The model under review builds one solid part; all positions refer to its coordinate system, in mm. Coordinates: 2 decimals unless noted, no trailing zeros. Order: outer loops, then holes, each group sorted by start corner. A loop starts at its lowest first (then second) coordinate and runs counter-clockwise, first axis right, second up. Notation, with made-up numbers: (66.5, -31) -> (104.5, -31) arc R13 cw to (104.5, -25) -> close; hole circle Ø3 at (18, -21.5). An arc over 180 degrees is marked (long way). Use one line per item in the form item = value. Start each with the question number.
(1) Take a section at A-A (z = 38). State the section outline as (x, y) points.
(2) Take a section at C-C (x = 4.75). State the section outline as (y, z) points, then the cut area to 3 significant figures.
(3) Insertion check: pin 1 Ø4 at (y, z) = (22.5, 85.5) entering from +X; pin 2 Ø2 at (x, y) = (4, -38.5) entering from -Z. Each pin has a flat end and moves straight along its axis. Give the tip position at first contact, or say it passes through.
(4) Take a section at B-B (y = -4.5). State the section outline as (x, z) points.
(5) Wall thickness on line 1 along X through (y, z) = (39.5, 91); line 2 along Z through (x, y) = (4, 18); line 3 along Z through (x, y) = (4.25, 23): over which ranges is each line inside the solid? List them lowest first.
```python
from build123d import *

# Parameters (mm, degrees)
F0_W        = 4.0632686578
F0_H        = 96.9379618764
F1_DEPTH    = 121
F2_W        = 94.1168889403
F2_H        = 118.3094680309
F3_DEPTH    = 0.2
F4_W        = 84.7520232201
F4_H        = 13.4229809046
F5_DEPTH    = 4.2
F6_T1_DEPTH = 109.4299485786
F6_T3_DEPTH = 38.1009062631


# Not quite as in the source:
# - a fillet or chamfer that OpenCascade refuses, or shapes differently, is made with other operations: its cross-section is extruded or revolved along the edge and cut away or added


with BuildPart() as f1:
    # F0 (on Top) → F1 (new body)
    with BuildSketch(Plane.XY):
        Rectangle(F0_W, F0_H)
    extrude(amount=F1_DEPTH)

    # F2 (on face) → F3 (join)
    with BuildSketch(Plane(origin=(-2.0316343289, 0, 0), x_dir=(0, -1, 0), z_dir=(-1, 0, 0))):
        with Locations((0, 60.4219585657)):
            Rectangle(F2_W, F2_H)
    extrude(amount=F3_DEPTH)

    # F4 (on face) → F5 (join)
    with BuildSketch(Plane.YZ.offset(2.0316343289)):
        with Locations((0, 111.4604696631)):
            Rectangle(F4_W, F4_H)
    extrude(amount=F5_DEPTH)

    # F6: fillet of radius 5 on 4 edges, made by hand

    # F6_s2 → F6_t1 (cut)
    with BuildSketch(Plane.XZ.offset(-54.7149742893)):
        with BuildLine():
            ThreePointArc((2.0316343289, 118.1719601154), (5.0395208818, 116.4767453929), (6.2316343289, 113.2363750437))
            Line((6.2316343289, 113.2363750437), (6.2316343289, 118.1719601154))
            Line((6.2316343289, 118.1719601154), (2.0316343289, 118.1719601154))
        make_face()
        with BuildLine():
            ThreePointArc((2.0316343289, 104.7489792109), (5.0395208818, 106.4441939334), (6.2316343289, 109.6845642826))
            Line((6.2316343289, 109.6845642826), (6.2316343289, 104.7489792109))
            Line((6.2316343289, 104.7489792109), (2.0316343289, 104.7489792109))
        make_face()
    extrude(amount=F6_T1_DEPTH, mode=Mode.SUBTRACT)

    # F6_s4 → F6_t3 (cut)
    with BuildSketch(Plane.XY.offset(92.4100165316)):
        with BuildLine():
            ThreePointArc((2.0316343289, -42.37601161), (5.0395208818, -40.6807968875), (6.2316343289, -37.4404265383))
            Line((6.2316343289, -37.4404265383), (6.2316343289, -42.37601161))
            Line((6.2316343289, -42.37601161), (2.0316343289, -42.37601161))
        make_face()
        with BuildLine():
            ThreePointArc((2.0316343289, 42.37601161), (5.0395208818, 40.6807968875), (6.2316343289, 37.4404265383))
            Line((6.2316343289, 37.4404265383), (6.2316343289, 42.37601161))
            Line((6.2316343289, 42.37601161), (2.0316343289, 42.37601161))
        make_face()
    extrude(amount=F6_T3_DEPTH, mode=Mode.SUBTRACT)


solid = f1.part
```
Findings:
q1.outline = (-2.23, -47.06) -> (-2.03, -47.06) -> (-2.03, -48.47) -> (2.03, -48.47) -> (2.03, 48.47) -> (-2.03, 48.47) -> (-2.03, 47.06) -> (-2.23, 47.06) -> close
q2.outline = (-40.99, 106.13) -> (40.99, 106.13) -> (40.99, 116.79) -> (-40.99, 116.79) -> close
q2.area = 874 mm²
q3.pin_1 = 2.03
q3.pin_2 = 105.01
q4.outline = (-2.23, 1.27) -> (-2.03, 1.27) -> (-2.03, 0) -> (2.03, 0) -> (2.03, 104.75) arc R5 ccw to (6.23, 109.68) -> (6.23, 113.24) arc R5 ccw to (2.03, 118.17) -> (2.03, 121) -> (-2.03, 121) -> (-2.03, 119.58) -> (-2.23, 119.58) -> close
q5.line_1 = -2.23 to 2.03
q5.line_2 = 105.52 to 117.4
q5.line_3 = 105.7 to 117.22
